Work out the finished part from the listing and answer in its coordinate system (mm). A direction names the side the tool comes from. Round coordinates to 2 decimals unless told otherwise and drop trailing zeros. Order: outer loops, then holes, each group sorted by start corner. A loop starts at its lowest first (then second) coordinate and runs counter-clockwise, first axis right, second up. Notation, with made-up numbers: (1, -13.75) -> (6, -13.75) arc R20 cw to (6, 18.25) -> close; hole circle Ø10 at (43.5, 4). An arc over 180 degrees is marked (long way). Use a Markdown table: item, result. Add a question column.
Item 1: A cutting plane is placed at B-B, the plane y = 15. Determine the outline of the cut face in (x, z), plus the area to 3 significant figures.
Item 2: Find the intervals of material crossed by L1, parallel to X at y = 0, z = -55.5; L2, parallel to X at y = 15, z = -55; L3, parallel to Y at x = 33, z = -61.75, in increasing order. Write a range as [from, to].
Item 3: Flat-ended cylindrical pins translate along their axes: P1, Ø5, axis at x = 11.25, y = 0, coming from the -Z side; P2, Ø8, axis at x = 5.5, y = -31.5, coming from the +Z side; P3, Ø6.5, axis at x = 0, y = -9.5, coming from the +Z side; P4, Ø4, axis at x = -15.5, y = -43.5, coming from the -Z side. Find the tip coordinate at first contact, or state that the pin passes through.
Item 4: A cutting plane is placed at A-A, the plane x = -32.5. Determine the outline of the cut face in (y, z), plus the area to 3 significant figures.
Item 5: For a pull along X with two mould halves and no side action, classify faces 4 (the flat face through (9, -15, -50)), 5 (the cylindrical face through (-1.375, 0.715, -57.409)), 6 (the cylindrical face through (-36.297, -48.859, -57.605)) as +X half, -X half, draft (parallel to the pull), parting line (faces both ways), or undercut.
Item 6: A tool of negligible diameter and unlimited length cuts with its end or side. For faces 1 (the flat face through (27.5, -44, -57)), 2 (the cylindrical face through (11.046, -35.042, -52.479)), 3 (the cylindrical face through (36.359, -48.797, -52.535)), from which of +Z, -Z, +X, -X, +Y, -Y can it reach the whole face along a straight path? Write none if from no direction.
from build123d import *

# Parameters (mm, degrees)
SKETCH007_W     = 70
SKETCH007_H     = 75
SKETCH007_R     = 6.1
SKETCH007_R_2   = 11.1
SKETCH007_R_3   = 2.05
SKETCH007_R_4   = 1.55
SKETCH007_R_5   = 2.55
PAD002_DEPTH    = 15
SKETCH008_R     = 13.1
POCKET004_DEPTH = 4
SKETCH009_R     = 13.1
POCKET005_DEPTH = 4
SKETCH010_R     = 2.20158
SKETCH010_R_2   = 2.512723
POCKET006_DEPTH = 10
SKETCH011_R     = 1.55
POCKET007_DEPTH = 15.001
CHAMFER003_SIZE = 1
CHAMFER004_SIZE = 1
CHAMFER005_SIZE = 1
FILLET_R        = 4


with BuildPart() as part:
    # Sketch007 (on Face1 of CopyChamfer002001) → Pad002 (new body)
    with BuildSketch(Plane.YX.offset(50)):
        with Locations((-15, 0)):
            Rectangle(SKETCH007_W, SKETCH007_H)
        with Locations((-33, 23)):
            Circle(SKETCH007_R, mode=Mode.SUBTRACT)
        with Locations((-33, -23)):
            Circle(SKETCH007_R, mode=Mode.SUBTRACT)
        with Locations((-28, 0)):
            Circle(SKETCH007_R_2, mode=Mode.SUBTRACT)
        with Locations((-46.5, 0)):
            Circle(SKETCH007_R_3, mode=Mode.SUBTRACT)
        with Locations((-9.5, 0)):
            Circle(SKETCH007_R_3, mode=Mode.SUBTRACT)
        with Locations((0, 22.5)):
            Circle(SKETCH007_R_4, mode=Mode.SUBTRACT)
        with Locations((0, 11.25)):
            Circle(SKETCH007_R_4, mode=Mode.SUBTRACT)
        Circle(SKETCH007_R_4, mode=Mode.SUBTRACT)
        with Locations((0, -11.25)):
            Circle(SKETCH007_R_4, mode=Mode.SUBTRACT)
        with Locations((0, -22.5)):
            Circle(SKETCH007_R_4, mode=Mode.SUBTRACT)
        with Locations((-15, 32.5)):
            Circle(SKETCH007_R_5, mode=Mode.SUBTRACT)
        with Locations((-15, -32.5)):
            Circle(SKETCH007_R_5, mode=Mode.SUBTRACT)
        with Locations((15, -32.5)):
            Circle(SKETCH007_R_5, mode=Mode.SUBTRACT)
        with Locations((15, 32.5)):
            Circle(SKETCH007_R_5, mode=Mode.SUBTRACT)
    extrude(amount=PAD002_DEPTH)

    # Sketch008 (on Face20 of Pad002) → Pocket004 (cut)
    with BuildSketch(Plane.YX.offset(65)):
        with Locations((-28, 0)):
            Circle(SKETCH008_R)
    extrude(amount=-POCKET004_DEPTH, mode=Mode.SUBTRACT)

    # Sketch009 (on Face4 of Pocket004) → Pocket005 (cut)
    with BuildSketch(Plane(origin=(0, 0, -50), x_dir=(0, -1, 0), z_dir=(0, 0, 1))):
        with Locations((28, 0)):
            Circle(SKETCH009_R)
    extrude(amount=-POCKET005_DEPTH, mode=Mode.SUBTRACT)

    # Sketch010 (on Face1 of Pocket005) → Pocket006 (cut)
    with BuildSketch(Plane.YZ.offset(37.5)):
        with Locations((-44, -57.5)):
            Circle(SKETCH010_R)
        with Locations((-32, -57.5)):
            Circle(SKETCH010_R_2)
    extrude(amount=-POCKET006_DEPTH, mode=Mode.SUBTRACT)

    # Sketch011 (on Face4 of Pocket006) → Pocket007 (cut, through all)
    with BuildSketch(Plane.YX.offset(65)):
        with Locations((-12.5, -15.5)):
            Circle(SKETCH011_R)
        with Locations((-12.5, 15.5)):
            Circle(SKETCH011_R)
        with Locations((-43.5, 15.5)):
            Circle(SKETCH011_R)
        with Locations((-43.5, -15.5)):
            Circle(SKETCH011_R)
    extrude(amount=-POCKET007_DEPTH, mode=Mode.SUBTRACT)

    # Chamfer003
    chamfer003_edges = [part.edges().sort_by_distance(p)[0] for p in [
        (-23, -39.1, -65),
        (23, -39.1, -65),
        (0, -41.1, -65),
        (32.5, -17.55, -65),
        (-32.5, -17.55, -65),
        (-32.5, 12.45, -65),
        (32.5, 12.45, -65),
        (22.5, -1.55, -65),
        (11.25, -1.55, -65),
        (0, -1.55, -65),
        (-11.25, -1.55, -65),
        (-22.5, -1.55, -65),
        (-15.5, -14.05, -65),
        (15.5, -14.05, -65),
        (15.5, -45.05, -65),
        (0, -48.55, -65),
        (-15.5, -45.05, -65),
        (0, -11.55, -65),
    ]]
    chamfer(chamfer003_edges, length=CHAMFER003_SIZE)

    # Chamfer004
    chamfer004_edges = [part.edges().sort_by_distance(p)[0] for p in [
        (-23, -39.1, -50),
        (-15.5, -45.05, -50),
        (0, -48.55, -50),
        (15.5, -45.05, -50),
        (23, -39.1, -50),
        (0, -14.9, -50),
        (32.5, -17.55, -50),
        (15.5, -14.05, -50),
        (23, -39.1, -64),
        (0, -1.55, -50),
        (-22.5, -1.55, -50),
        (-11.25, -1.55, -50),
        (-15.5, -14.05, -50),
        (0, -11.55, -50),
        (11.25, -1.55, -50),
        (22.5, -1.55, -50),
        (32.5, 12.45, -50),
        (-32.5, -17.55, -50),
        (-32.5, 12.45, -50),
    ]]
    chamfer(chamfer004_edges, length=CHAMFER004_SIZE)

    # Chamfer005
    chamfer005_edges = [part.edges().sort_by_distance(p)[0] for p in [
        (37.5, -34.512723, -57.5),
        (37.5, -46.20158, -57.5),
    ]]
    chamfer(chamfer005_edges, length=CHAMFER005_SIZE)

    # Fillet
    fillet_edges = [part.edges().sort_by_distance(p)[0] for p in [
        (37.5, 20, -57.5),
        (37.5, -50, -57.5),
        (-37.5, 20, -57.5),
        (-37.5, -50, -57.5),
    ]]
    fillet(fillet_edges, radius=FILLET_R)


solid = part.part
Reported:
| question | item | result |
|---|---|---|
| 1 | outline | (-37.5, -65) -> (-36.05, -65) -> (-35.05, -64) -> (-35.05, -51) -> (-36.05, -50) -> (-37.5, -50) -> close; (-29.95, -64) -> (-28.95, -65) -> (28.95, -65) -> (29.95, -64) -> (29.95, -51) -> (28.95, -50) -> (-28.95, -50) -> (-29.95, -51) -> close; (35.05, -64) -> (36.05, -65) -> (37.5, -65) -> (37.5, -50) -> (36.05, -50) -> (35.05, -51) -> close |
| 1 | area | 968 mm² |
| 2 | L1 | [-37.5, -24.05], [-20.95, -12.8], [-9.7, -1.55], [1.55, 9.7], [12.8, 20.95], [24.05, 37.5] |
| 2 | L2 | [-37.5, -35.05], [-29.95, 29.95], [35.05, 37.5] |
| 2 | L3 | [-50, -17.5], [-12.5, 12.5], [17.5, 20] |
| 3 | P1 | z = -64.95 |
| 3 | P2 | through |
| 3 | P3 | z = -50 |
| 3 | P4 | z = -64.45 |
| 4 | outline | (-50, -65) -> (-18.55, -65) -> (-17.55, -64) -> (-17.55, -51) -> (-18.55, -50) -> (-50, -50) -> close; (-12.45, -64) -> (-11.45, -65) -> (11.45, -65) -> (12.45, -64) -> (12.45, -51) -> (11.45, -50) -> (-11.45, -50) -> (-12.45, -51) -> close; (17.55, -64) -> (18.55, -65) -> (20, -65) -> (20, -50) -> (18.55, -50) -> (17.55, -51) -> close |
| 4 | area | 893 mm² |
| 5 | face 4 | draft |
| 5 | face 5 | undercut |
| 5 | face 6 | -X half |
| 6 | face 1 | +X |
| 6 | face 2 | +Z |
| 6 | face 3 | +Z, +X, -Y |
